```python
from build123d import *

# Parameters (mm, degrees)
BOSS_EXTRUDE1_DEPTH = 76.2
SKETCH2_R           = 3.175
CUT_EXTRUDE1_DEPTH  = 154.932715085


with BuildPart() as part:
    # Sketch1 → Boss-Extrude1 (new body)
    with BuildSketch(Plane.XY):
        with BuildLine():
            Line((-12.7, 113.592253257), (-14.829854749, 132.642253257))
            Line((-14.829854749, 132.642253257), (-12.305582454, 132.924475479))
            Line((-12.305582454, 132.924475479), (-10.454881932, 116.371306789))
            ThreePointArc((-10.454881932, 116.371306789), (1.128111355, 116.834553813), (12.7, 116.14773179))
            Line((12.7, 116.14773179), (12.7, 113.592253257))
            ThreePointArc((12.7, 113.592253257), (0, 114.3), (-12.7, 113.592253257))
        make_face()
    extrude(amount=BOSS_EXTRUDE1_DEPTH)

    # Sketch2 → Cut-Extrude1 (cut, through all)
    with BuildSketch(Plane(origin=(0, 0, 0), x_dir=(1, 0, 0), z_dir=(0, 1, 0))):
        with Locations(Location((0, -12.7, 0), (0, 0, 90))):
            Circle(SKETCH2_R)
        with Locations(Location((0, -63.5, 0), (0, 0, 90))):
            Circle(SKETCH2_R)
    extrude(amount=CUT_EXTRUDE1_DEPTH, mode=Mode.SUBTRACT)


solid = part.part
```
Can you work these out from the model? Positions are in its coordinate system, mm. Round coordinates to 2 decimals unless told otherwise and drop trailing zeros. Loops run counter-clockwise (first coordinate to the right, second up) from the corner with the lowest first, then second, coordinate; pieces in that order, holes last.
Item 1: Suppose I cut it at C-C, the plane z = 27.5. Write out the boundary of the cut face in (x, y).
Item 2: Please list where these lines run through material, in increasing order: L1, parallel to X at y = 115.45, z = 12.7 (3 decimals); L2, parallel to Y at x = -1, z = 47; L3, parallel to X at y = 121.5, z = 22.5.
Item 3: Suppose I cut it at B-B, the plane z = 63.5. Write out the boundary of the cut face in (x, y) (3 decimals), then the cut area to 3 significant figures.
Item 4: Will these pins go through, and if not, where does the flat tip stop? pin 1 Ø1 at (x, z) = (-3.5, 42) entering from +Y; pin 2 Ø5 at (y, z) = (120, 40.5) entering from -X; pin 3 Ø10 at (y, z) = (119.5, 35.5) entering from -X; pin 4 Ø5.5 at (x, z) = (0, 12.7) entering from -Y.
Item 5: If we mould it in two halves opening along X, with no side actions, what happens to faces 1 (the cylindrical face through (0.966, 116.836, 37.567)), 2 (the cylindrical face through (0.2, 114.3, 37.6)), 3 (the flat face through (-5, 116, 76.2)), 4 (the flat face through (12.7, 115, 38))? For each: +X half, -X half, draft (parallel to the pull), parting line (faces both ways), or undercut.
Item 6: Suppose I cut it at D-D, the plane x = 6. Write out the boundary of the cut face in (y, z).
Item 7: Suppose I cut it at A-A, the plane x = 0. Write out the boundary of the cut face in (y, z) (3 decimals), then the cut area to 3 significant figures.
Reported:
1. outline: (-14.83, 132.64) - (-12.7, 113.59) arc R114.3 cw to (12.7, 113.59) - (12.7, 116.15) arc R116.84 ccw to (-10.45, 116.37) - (-12.31, 132.92) - close
2. L1: x = -12.908 to -3.175, 3.175 to 12.7
2. L2: y = 114.3 to 116.84
2. L3: x = -13.58 to -11.03
3. outline: (-14.83, 132.642) - (-12.7, 113.592) arc R114.3 cw to (-3.175, 114.256) - (-3.175, 116.797) arc R116.84 ccw to (-10.455, 116.371) - (-12.306, 132.924) - close; (3.175, 114.256) arc R114.3 cw to (12.7, 113.592) - (12.7, 116.148) arc R116.84 ccw to (3.175, 116.797) - close
3. area: 91.1 mm2
4. pin 1: stops at y = 116.8
4. pin 2: stops at x = -13.7
4. pin 3: stops at x = -13.92
4. pin 4: passes through
5. face 1: undercut
5. face 2: undercut
5. face 3: draft
5. face 4: +X half
6. outline: (114.14, 0) - (116.69, 0) - (116.69, 76.2) - (114.14, 76.2) - close
7. outline: (114.3, 0) - (116.84, 0) - (116.84, 9.525) - (114.3, 9.525) - close; (114.3, 15.875) - (116.84, 15.875) - (116.84, 60.325) - (114.3, 60.325) - close; (114.3, 66.675) - (116.84, 66.675) - (116.84, 76.2) - (114.3, 76.2) - close
7. area: 161 mm2
